Autodesk Inventor part; units mm, degrees
ref_plane "YZ Plane" through (0, 0, 0) normal (1, 0, 0) x (0, 1, 0)
ref_plane "XZ Plane" through (0, 0, 0) normal (0, 1, 0) x (-1, 0, 0)
ref_plane "XY Plane" through (0, 0, 0) normal (0, 0, 1) x (1, 0, 0)
sketch "Sketch2" plane through (0, 0, 0) normal (0, 1, 0) x (-1, 0, 0)
  line L0 (0, 0) -> (-101.6, 0)
  line L1 (-101.6, 0) -> (-101.6, -127)
  line L2 (-101.6, -127) -> (0, -127)
  line L3 (0, -127) -> (0, 0)
  dimension "d0" = 127
  dimension "d1" = 101.6
extrude "Extrusion1" add sketch "Sketch2" along normal blind 3.175
sketch "Sketch3" plane through (0, 3.175, 0) normal (0, 1, 0) x (1, 0, 0)
  line L0 (101.6, 127) -> (0, 127)
  line L1 (35.12, 112.2299) -> (63.5, 14.7782)
  line L2 (63.5, 14.7782) -> (91.88, 112.2299)
  line L3 (0, 127) -> (0, 0)
  line L4 (0, 0) -> (101.6, 0)
  dimension "d5" = 14.7701
  dimension "d6" = 14.7701
  dimension "d9" = 56.76
  dimension "d27" = 101.5
  dimension "d28" = 101.5
  dimension "d58" = 63.5
  dimension "d60" = 97.4517
  dimension "d61" = 14.7782
hole "Hole1" at (35.12, 3.175, -112.2299) at (91.88, 3.175, -112.2299) at (63.5, 3.175, -14.7782) direction (0, -1, 0) diameter 5 end through all
sketch "Sketch5" plane through (0, 0, 0) normal (0, -1, 0) x (1, 0, 0)
  circle A0 centre (91.88, -112.2299) radius 2.5
  circle A1 centre (35.12, -112.2299) radius 2.5
  line L0 (63.5, -63.1355) -> (91.88, -112.2299)
  line L1 (33.5, -93.1355) -> (93.5, -93.1355)
  line L2 (93.5, -93.1355) -> (93.5, -33.1355)
  line L3 (93.5, -33.1355) -> (33.5, -33.1355)
  line L4 (33.5, -33.1355) -> (33.5, -93.1355)
  line L5 (33.5, -93.1355) -> (93.5, -33.1355) construction
  line L6 (93.5, -93.1355) -> (33.5, -33.1355) construction
  dimension "d33" = 56.707
  dimension "d34" = 56.707
  dimension "d56" = 60
  dimension "d57" = 60
extrude "Extrusion2" cut sketch "Sketch5" against normal blind 25.4 contours L1 L4 L3 L2
sketch "Sketch6" plane through (101.6, 0, 0) normal (1, 0, 0) x (0, 0, -1)
  line L0 (0, 0) -> (127, 0)
  line L1 (127, 0) -> (127, 3.175)
  line L2 (0, 0) -> (127, 0)
  line L3 (127, 0) -> (127, 3.175)
  line L4 (127, 3.175) -> (0, 3.175)
  line L5 (0, 3.175) -> (0, 0)
extrude "Extrusion3" add sketch "Sketch6" along normal blind 25.4
sketch "Sketch7" plane through (0, 3.175, 0) normal (0, 1, 0) x (1, 0, 0)
  line L0 (0, 0) -> (127, 0)
  line L1 (127, 127) -> (127, 0)
  line L2 (0, 127) -> (127, 127)
  line L3 (0, 127) -> (0, 0)
  point P0 (12.7, 63.5)
  point P1 (114.3, 114.3)
  point P2 (114.3, 12.7)
  point P3 (12.7, 12.7)
  dimension "d39" = 63.5
  dimension "d40" = 12.7
  dimension "d41" = 12.7
  dimension "d42" = 12.7
  dimension "d43" = 12.7
  dimension "d44" = 12.7
  dimension "d45" = 12.7
  dimension "d46" = 113.5923
  dimension "d47" = 101.6
  dimension "d48" = 50.8
  dimension "d59" = 101.6
hole "Hole2" at (12.7, 3.175, -63.5) at (114.3, 3.175, -114.3) at (114.3, 3.175, -12.7) at (12.7, 3.175, -12.7) direction (0, -1, 0) diameter 6.35 end through all
properties part number "Window_MotorMounting" material "Aluminum 6061"
Input: part model. Units: mm. Frame: model coordinates. A direction names the side the tool comes from. Coordinates: 2 decimals unless noted, no trailing zeros. Order: outer loops, then holes, each group sorted by start corner. A loop starts at its lowest first (then second) coordinate and runs counter-clockwise, first axis right, second up. Notation, with made-up numbers: M 71,22.5 L 95,22.5 A37 cw 95,61.5 Z; hole C 13.25,87 d7. An arc over 180 degrees is marked long. One line per question, with ' | ' between items.
Item 1: Ray query, line 1 along Z through (x, y) = (114.3, 1.25) (3 decimals); line 2 along Z through (x, y) = (63.5, 0.9); line 3 along X through (y, z) = (1.3, -93). Return the intervals inside material, ascending.
Geometry results:
line 1: z = -127 to -117.475, -111.125 to -15.875, -9.525 to 0 | line 2: z = -127 to -93.14, -33.14 to -17.28, -12.28 to 0 | line 3: x = 0 to 33.5, 93.5 to 127
Item 2: Draft query along X for faces 1 (the flat face through (63, 2, 0)), 2 (the cylindrical face through (64.46, 1.57, -12.47)), 3 (the flat face through (127, 2, -63)). Return one class per face: released by +X, released by -X, zero draft, split by the parting line, or undercut.
Geometry results:
face 1: zero draft | face 2: undercut | face 3: released by +X
Item 3: Section A-A (x = 35.12). Output: boundary loops of the cut face in (y, z) (1 decimal).
Geometry results:
outline: M 0,-127 L 3.2,-127 L 3.2,-114.7 L 0,-114.7 Z; M 0,-109.7 L 3.2,-109.7 L 3.2,-93.1 L 0,-93.1 Z; M 0,-33.1 L 3.2,-33.1 L 3.2,0 L 0,0 Z
Item 4: Section D-D (y = 2.15). Give the number of separate pieces and of enclosed holes in the cut face, then the cut area to 3 significant figures.
Geometry results:
separate pieces: 1 | enclosed holes: 8 | area: 12,300 mm^2
Item 5: Reachability of faces 4 (the flat face through (0, 2, -64)), 5 (the flat face through (64, 2, -33.136)) from +Z, -Z, +X, -X, +Y, -Y: full face, straight path, thin tool, end or side. Return the list, or none.
Geometry results:
face 4: +Z, -Z, -X, +Y, -Y | face 5: +Y, -Y
Item 6: Section C-C (x = 49). Output: boundary loops of the cut face in (y, z) (1 decimal).
Geometry results:
outline: M 0,-127 L 3.2,-127 L 3.2,-93.1 L 0,-93.1 Z; M 0,-33.1 L 3.2,-33.1 L 3.2,0 L 0,0 Z
Item 7: Section B-B (z = -86). Output: boundary loops of the cut face in (x, y) (3 decimals), then the cut area to 3 significant figures.
Geometry results:
outline: M 0,0 L 33.5,0 L 33.5,3.175 L 0,3.175 Z; M 93.5,0 L 127,0 L 127,3.175 L 93.5,3.175 Z | area: 213 mm^2
